Design review of the part built by this model. Coordinates are the model's own, in mm. Coordinates: 2 decimals unless noted, no trailing zeros. Order: outer loops, then holes, each group sorted by start corner. A loop starts at its lowest first (then second) coordinate and runs counter-clockwise, first axis right, second up. Notation, with made-up numbers: (27.5, -1) -> (78.5, -1) arc R14 ccw to (78.5, 7) -> close; hole circle Ø11 at (46.5, 11.5). An arc over 180 degrees is marked (long way). Use a Markdown table: item, result. Add a question column.
Q1. Wall thickness on probe 1 along Y at (x, z) = (42, 2.5); probe 2 along Y at (x, z) = (11, 5.75); probe 3 along Z at (x, y) = (7, 27): over which ranges is each line inside the solid? List them lowest first.
Q2. Add section A-A (z = 8). State the section outline as (x, y) points, then the cut area to 3 significant figures.
Q3. Add section C-C (x = -3). State the section outline as (y, z) points.
Q4. Insertion check: pin 1 (4 mm diameter, centred on y = 41.5, z = 10, fed in from +X); pin 2 (3 mm diameter, centred on y = 20.5, z = 9, fed in from +X); pin 3 (5 mm diameter, centred on y = 32, z = 10, fed in from -X). Each pin has a flat end and moves straight along its axis. Give the tip position at first contact, or say it passes through.
Q5. Add section B-B (x = 35). State the section outline as (y, z) points, then the cut area to 3 significant figures.
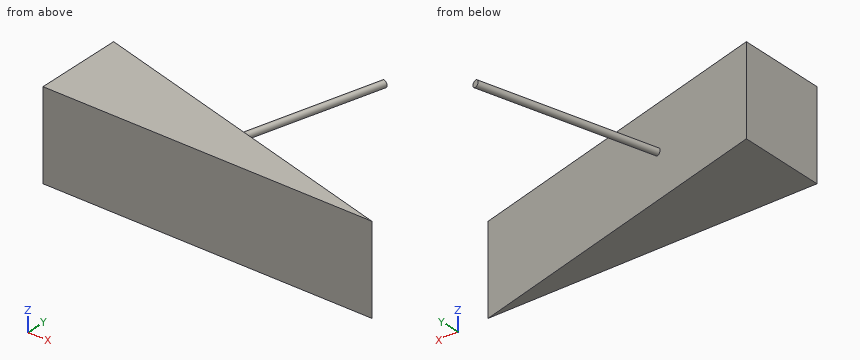
from build123d import *

# Parameters (mm, degrees)
BOSS_EXTRUDE1_DEPTH = 20
SKETCH2_R           = 0.75
BOSS_EXTRUDE2_DEPTH = 40


with BuildPart() as part:
    # Sketch1 → Boss-Extrude1 (new body)
    with BuildSketch(Plane.XY):
        Polygon((-22.150682767, 20), (52.490333384, 0), (-22.150682767, 0), align=None)
    extrude(amount=BOSS_EXTRUDE1_DEPTH)

    # Sketch2 → Boss-Extrude2 (add)
    with BuildSketch(Plane(origin=(3.51618561, 13.122583346, 0), x_dir=(0.96592582628907, -0.25881904510251424, 0), z_dir=(0.2588190451025143, 0.9659258262890701, 0))):
        with Locations((0, -10)):
            Circle(SKETCH2_R)
    extrude(amount=BOSS_EXTRUDE2_DEPTH)


solid = part.part
Established:
| question | item | result |
|---|---|---|
| 1 | probe 1 | 0 to 2.81 |
| 1 | probe 2 | 0 to 11.12 |
| 1 | probe 3 | 9.29 to 10.71 |
| 2 | outline | (-22.15, 0) -> (52.49, 0) -> (-22.15, 20) -> close |
| 2 | area | 746 mm^2 |
| 3 | outline | (0, 0) -> (14.87, 0) -> (14.87, 20) -> (0, 20) -> close |
| 4 | pin 1 | x = 12.43 |
| 4 | pin 2 | x = 6.59 |
| 4 | pin 3 | x = 7.13 |
| 5 | outline | (0, 0) -> (4.69, 0) -> (4.69, 20) -> (0, 20) -> close |
| 5 | area | 93.7 mm^2 |
